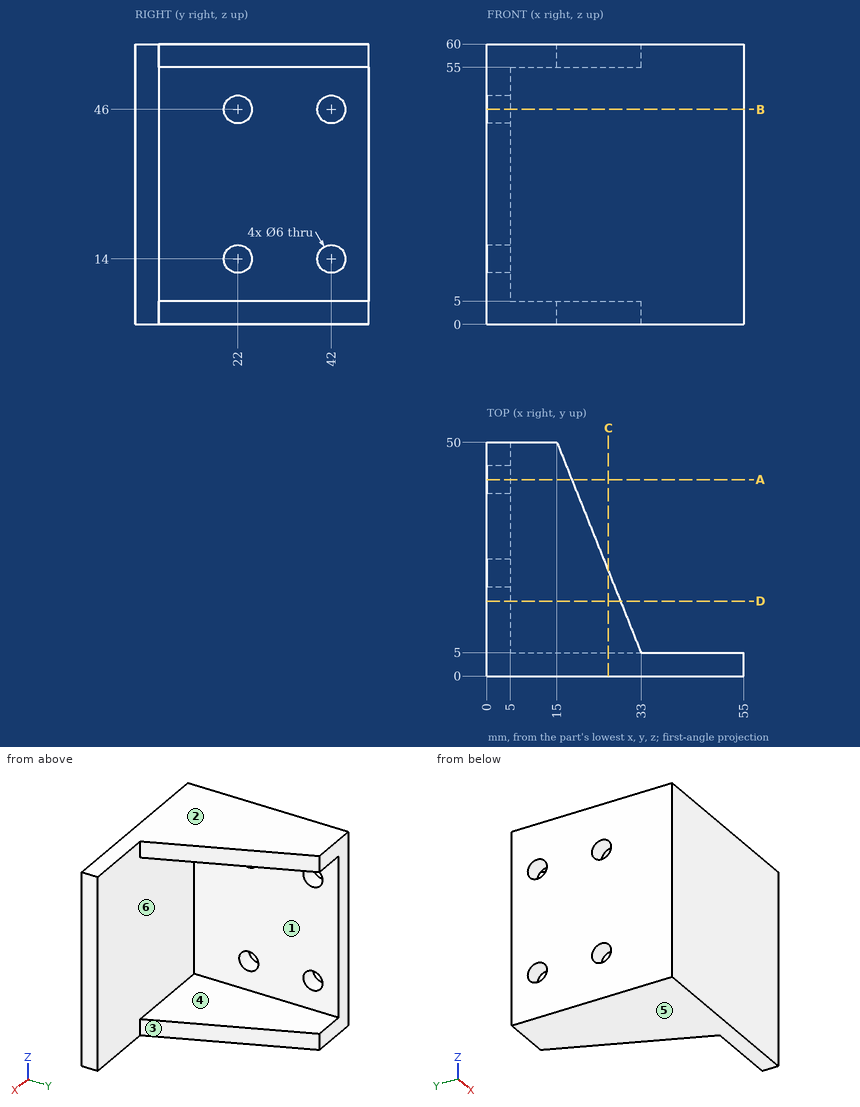
Answer from the drawing. Dimensions are ordinates in mm from the lowest x, y and z of the part. A direction names the side the tool comes from. Round coordinates to 2 decimals unless told otherwise and drop trailing zeros. Loops run counter-clockwise (first coordinate to the right, second up) from the corner with the lowest first, then second, coordinate; pieces in that order, holes last.
Q1. Section B-B on z = 46 is taken. Write down the section's boundary in (x, y), and give its area (3 significant figures).
Q2. Consider probe 1 along Y at (x, z) = (3.1, 46); probe 2 along Z at (x, y) = (24.5, 8); probe 3 along Y at (x, z) = (36, 44). Determine where each line is inside the solid, lowest interval first.
Q3. Which of the six approach directions +Z, -Z, +X, -X, +Y, -Y give full straight-line access (tool end or side, diameter ignored) to the marked faces 1 and 2?
Q4. Each of these flat-tipped pins is pushed along its axis until it touches: pin 1 (8 mm diameter, centred on y = 43, z = 26, fed in from +X); pin 2 (5.5 mm diameter, centred on y = 42, z = 46, fed in from +X); pin 3 (3 mm diameter, centred on x = 44, z = 17, fed in from +Y). Where does it stop, or does it pass through?
Q5. Determine the mould class of the marked faces 3, 4, 5 and 6 for opening direction Z: released by +Z, released by -Z, zero draft, split by the parting line, or undercut.
Q6. Section C-C on x = 26 is taken. Write down the section's boundary in (y, z).
Q7. Section D-D on y = 16 is taken. Write down the section's boundary in (x, z).
Q8. Section A-A on y = 42 is taken. Write down the section's boundary in (x, z).
Output:
1. outline: (0, 0) - (55, 0) - (55, 5) - (5, 5) - (5, 19) - (0, 19) - close; (0, 25) - (5, 25) - (5, 39) - (0, 39) - close; (0, 45) - (5, 45) - (5, 50) - (0, 50) - close
1. area: 440 mm2
2. probe 1: y = 0 to 19, 25 to 39, 45 to 50
2. probe 2: z = 0 to 5, 55 to 60
2. probe 3: y = 0 to 5
3. face 1: +X, +Y
3. face 2: +Z, +X, -X, +Y, -Y
4. pin 1: stops at x = 5
4. pin 2: passes through
4. pin 3: stops at y = 5
5. face 3: zero draft
5. face 4: undercut
5. face 5: released by -Z
5. face 6: undercut
6. outline: (0, 0) - (22.5, 0) - (22.5, 5) - (5, 5) - (5, 55) - (22.5, 55) - (22.5, 60) - (0, 60) - close
7. outline: (0, 0) - (28.6, 0) - (28.6, 5) - (5, 5) - (5, 55) - (28.6, 55) - (28.6, 60) - (0, 60) - close
8. outline: (0, 0) - (18.2, 0) - (18.2, 5) - (5, 5) - (5, 11) - (0, 11) - close; (0, 17) - (5, 17) - (5, 43) - (0, 43) - close; (0, 49) - (5, 49) - (5, 55) - (18.2, 55) - (18.2, 60) - (0, 60) - close
